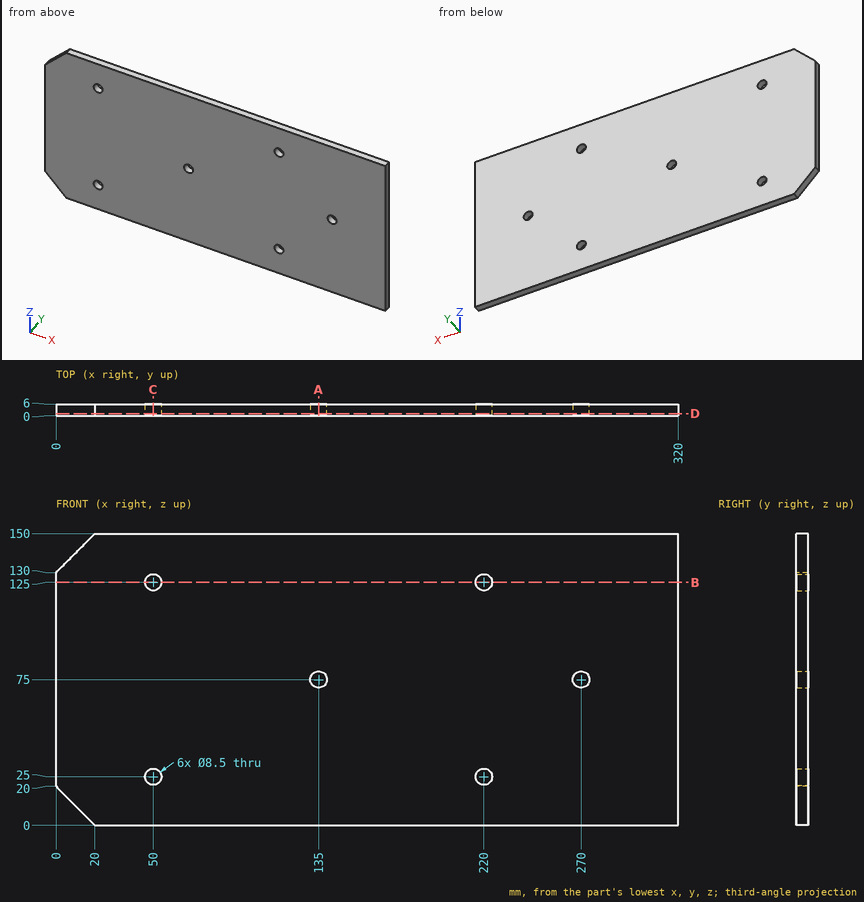
Answer from the drawing. Dimensions are ordinates in mm from the lowest x, y and z of the part. Coordinates: 2 decimals unless noted, no trailing zeros. Loops run counter-clockwise (first coordinate to the right, second up) from the corner with the lowest first, then second, coordinate; pieces in that order, holes last. Notation, with made-up numbers: (55, 9.5) -> (107, 9.5) arc R16 ccw to (107, 39.5) -> close; hole circle Ø3 at (72.25, 15). An arc over 180 degrees is marked (long way). Answer in a Markdown table with one row per item.
Item 1: A cutting plane is placed at B-B on z = 125. Determine the outline of the cut face in (x, y), plus the area to 3 significant figures.
Returned:
| item | result |
|---|---|
| outline | (0, 0) -> (45.75, 0) -> (45.75, 6) -> (0, 6) -> close; (54.25, 0) -> (215.75, 0) -> (215.75, 6) -> (54.25, 6) -> close; (224.25, 0) -> (320, 0) -> (320, 6) -> (224.25, 6) -> close |
| area | 1,820 mm^2 |
Item 2: A cutting plane is placed at D-D on y = 1. Determine the outline of the cut face in (x, z), plus the area to 3 significant figures.
Returned:
| item | result |
|---|---|
| outline | (0, 20) -> (20, 0) -> (320, 0) -> (320, 150) -> (20, 150) -> (0, 130) -> close; hole circle Ø8.5 at (50, 25); hole circle Ø8.5 at (50, 125); hole circle Ø8.5 at (135, 75); hole circle Ø8.5 at (220, 25); hole circle Ø8.5 at (220, 125); hole circle Ø8.5 at (270, 75) |
| area | 47,300 mm^2 |
Item 3: Straight lines are drawn through the part: line 1 along Z through (x, y) = (220, 1.9); line 2 along X through (y, z) = (5.75, 26); line 3 along Z through (x, y) = (135, 2.15). For each, find the intervals that lie inside material, in ascending order. Write a range as [from, to].
Returned:
| item | result |
|---|---|
| line 1 | z = [0, 20.75], [29.25, 120.75], [129.25, 150] |
| line 2 | x = [0, 45.87], [54.13, 215.87], [224.13, 320] |
| line 3 | z = [0, 70.75], [79.25, 150] |
Item 4: A cutting plane is placed at C-C on x = 50. Determine the outline of the cut face in (y, z), plus the area to 3 significant figures.
Returned:
| item | result |
|---|---|
| outline | (0, 0) -> (6, 0) -> (6, 20.75) -> (0, 20.75) -> close; (0, 29.25) -> (6, 29.25) -> (6, 120.75) -> (0, 120.75) -> close; (0, 129.25) -> (6, 129.25) -> (6, 150) -> (0, 150) -> close |
| area | 798 mm^2 |
Item 5: A cutting plane is placed at A-A on x = 135. Determine the outline of the cut face in (y, z), plus the area to 3 significant figures.
Returned:
| item | result |
|---|---|
| outline | (0, 0) -> (6, 0) -> (6, 70.75) -> (0, 70.75) -> close; (0, 79.25) -> (6, 79.25) -> (6, 150) -> (0, 150) -> close |
| area | 849 mm^2 |
